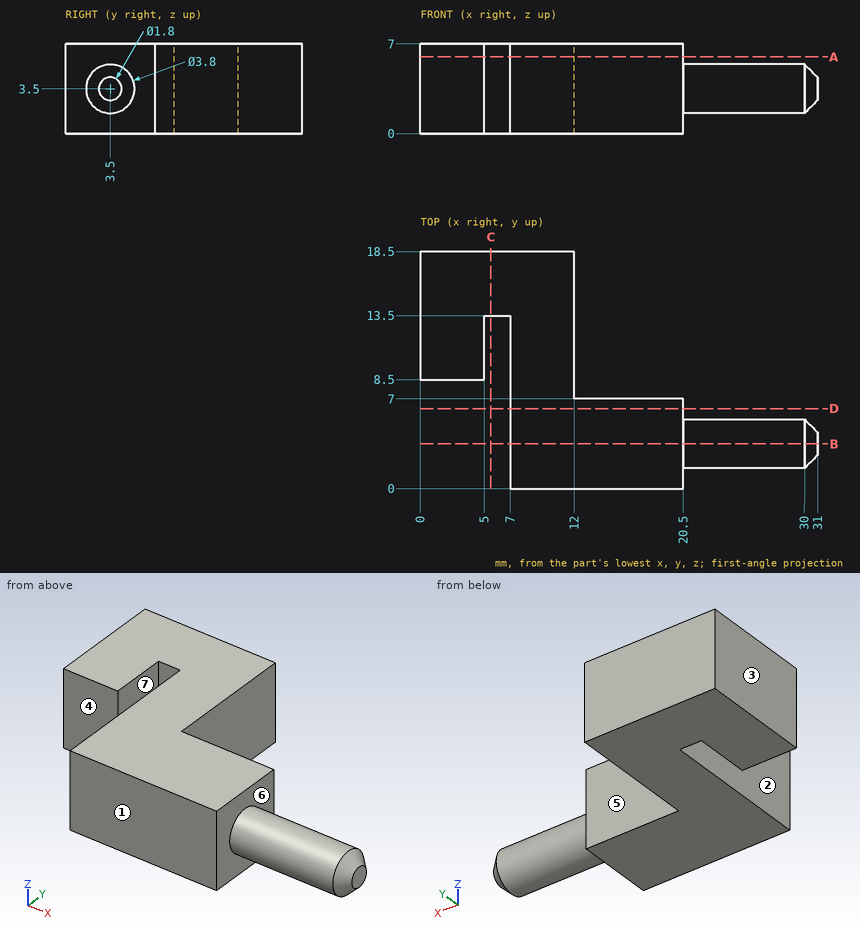
Part print with two shaded views. Sizes in mm from the minimum x, y, z corner. A direction names the side the tool comes from. Coordinates: 2 decimals unless noted, no trailing zeros. Loops run counter-clockwise (first coordinate to the right, second up) from the corner with the lowest first, then second, coordinate; pieces in that order, holes last. Notation, with made-up numbers: (10.5, 65) - (38.5, 65) arc R21 cw to (38.5, 85) - close; hole circle Ø10 at (31, 28.5). An arc over 180 degrees is marked (long way). Write each question's results on one line, items separated by ' | '. Start each with the question number.
Q1. Slice it at A-A on z = 6. Give the cut face in (x, y), and give its area (3 significant figures).
Q2. Slice it at C-C on x = 5.5. Give the cut face in (y, z).
Q3. Which spindle directions (+Z, -Z, +X, -X, +Y, -Y) get a long thin tool onto all of the face, cutting with end or side? Do the marked faces 4, 5, 6 and 7. Say none if no direction does.
Q4. Two-plate mould, pull along X, no slides. Class the marked faces 1, 2 and 3: +X half, -X half, draft (parallel to the pull), parting line (faces both ways), or undercut.
Q5. Slice it at B-B on y = 3.5. Give the cut face in (x, z), and give its area (3 significant figures).
Q6. Probe line 1 along X through (y, z) = (11, 1.75); line 2 along Y through (x, z) = (6.5, 5.25); line 3 along X through (y, z) = (7.5, 3.5). List the from-to ranges inside material, lowest first.
Q7. Slice it at D-D on y = 6.25. Give the cut face in (x, z), and give its area (3 significant figures).
Q8. Drop flat-ended pins along their axis: pin 1 Ø0.6 at (x, z) = (6, 2.5) entering from -Y; pin 2 Ø4 at (x, z) = (2, 4) entering from -Y; pin 3 Ø1.5 at (y, z) = (9, 4) entering from +X; pin 4 Ø4 at (x, z) = (8.5, 4) entering from -Y. Give the stop position or say it passes through.
Answer:
1) outline: (0, 8.5) - (5, 8.5) - (5, 13.5) - (7, 13.5) - (7, 0) - (20.5, 0) - (20.5, 7) - (12, 7) - (12, 18.5) - (0, 18.5) - close | area: 212 mm2
2) outline: (13.5, 0) - (18.5, 0) - (18.5, 7) - (13.5, 7) - close
3) face 4: +Z, -Z, -X, -Y | face 5: +Z, -Z, +X, +Y | face 6: +X | face 7: +Z, -Z, -Y
4) face 1: draft | face 2: undercut | face 3: -X half
5) outline: (7, 0) - (20.5, 0) - (20.5, 1.6) - (30, 1.6) - (31, 2.6) - (31, 4.4) - (30, 5.4) - (20.5, 5.4) - (20.5, 7) - (7, 7) - close | area: 133 mm2
6) line 1: x = 0 to 5, 7 to 12 | line 2: y = 13.5 to 18.5 | line 3: x = 7 to 12
7) outline: (7, 0) - (20.5, 0) - (20.5, 7) - (7, 7) - close | area: 94.5 mm2
8) pin 1: stops at y = 13.5 | pin 2: stops at y = 8.5 | pin 3: stops at x = 12 | pin 4: stops at y = 0
